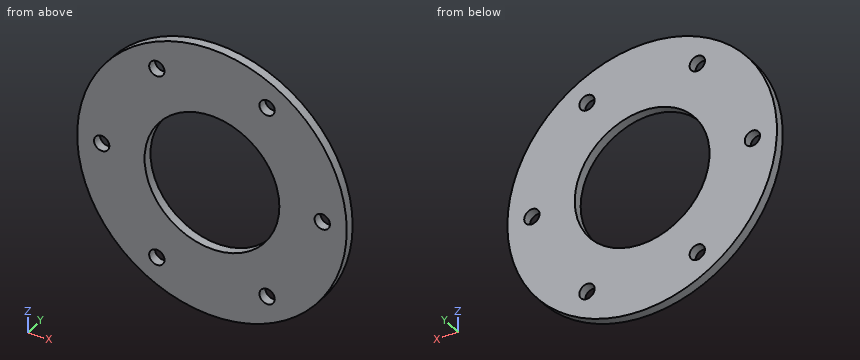
```python
from build123d import *

# Parameters (mm, degrees)
SKETCH1_R           = 139.7
SKETCH1_R_2         = 69.85
BOSS_EXTRUDE1_DEPTH = 9.525
CUT_EXTRUDE1_REACH  = 11.525
SKETCH2_R           = 7.9375


with BuildPart() as part:
    # Sketch1 → Boss-Extrude1 (new body)
    with BuildSketch(Plane(origin=(0, 0, 0), x_dir=(1, 0, 0), z_dir=(0, 1, 0))):
        with Locations((-63.18889636, 128.089070316)):
            Circle(SKETCH1_R)
        with Locations((-63.18889636, 128.089070316)):
            Circle(SKETCH1_R_2, mode=Mode.SUBTRACT)
    extrude(amount=BOSS_EXTRUDE1_DEPTH)

    # Sketch2 → Cut-Extrude1 (cut, up to next)
    with BuildSketch(Plane(origin=(0, 9.525, 0), x_dir=(1, 0, 0), z_dir=(0, 1, 0)), mode=Mode.PRIVATE) as cut_extrude1_sk1:
        with Locations((51.11110364, 128.089070316)):
            Circle(SKETCH2_R)
    cut_extrude1_tool1 = extrude(cut_extrude1_sk1.sketch, amount=-CUT_EXTRUDE1_REACH, mode=Mode.PRIVATE) & part.part
    add(cut_extrude1_tool1.solids().sort_by_distance((51.111104, 9.525, -128.08907))[0], mode=Mode.SUBTRACT)
    # Sketch2 → Cut-Extrude1 (cut, up to next)
    with BuildSketch(Plane(origin=(0, 9.525, 0), x_dir=(1, 0, 0), z_dir=(0, 1, 0)), mode=Mode.PRIVATE) as cut_extrude1_sk2:
        with Locations((-6.03889636, 227.075773969)):
            Circle(SKETCH2_R)
    cut_extrude1_tool2 = extrude(cut_extrude1_sk2.sketch, amount=-CUT_EXTRUDE1_REACH, mode=Mode.PRIVATE) & part.part
    add(cut_extrude1_tool2.solids().sort_by_distance((-6.038896, 9.525, -227.075774))[0], mode=Mode.SUBTRACT)
    # Sketch2 → Cut-Extrude1 (cut, up to next)
    with BuildSketch(Plane(origin=(0, 9.525, 0), x_dir=(1, 0, 0), z_dir=(0, 1, 0)), mode=Mode.PRIVATE) as cut_extrude1_sk3:
        with Locations((-120.33889636, 227.075773969)):
            Circle(SKETCH2_R)
    cut_extrude1_tool3 = extrude(cut_extrude1_sk3.sketch, amount=-CUT_EXTRUDE1_REACH, mode=Mode.PRIVATE) & part.part
    add(cut_extrude1_tool3.solids().sort_by_distance((-120.338896, 9.525, -227.075774))[0], mode=Mode.SUBTRACT)
    # Sketch2 → Cut-Extrude1 (cut, up to next)
    with BuildSketch(Plane(origin=(0, 9.525, 0), x_dir=(1, 0, 0), z_dir=(0, 1, 0)), mode=Mode.PRIVATE) as cut_extrude1_sk4:
        with Locations((-177.48889636, 128.089070316)):
            Circle(SKETCH2_R)
    cut_extrude1_tool4 = extrude(cut_extrude1_sk4.sketch, amount=-CUT_EXTRUDE1_REACH, mode=Mode.PRIVATE) & part.part
    add(cut_extrude1_tool4.solids().sort_by_distance((-177.488896, 9.525, -128.08907))[0], mode=Mode.SUBTRACT)
    # Sketch2 → Cut-Extrude1 (cut, up to next)
    with BuildSketch(Plane(origin=(0, 9.525, 0), x_dir=(1, 0, 0), z_dir=(0, 1, 0)), mode=Mode.PRIVATE) as cut_extrude1_sk5:
        with Locations((-120.33889636, 29.102366663)):
            Circle(SKETCH2_R)
    cut_extrude1_tool5 = extrude(cut_extrude1_sk5.sketch, amount=-CUT_EXTRUDE1_REACH, mode=Mode.PRIVATE) & part.part
    add(cut_extrude1_tool5.solids().sort_by_distance((-120.338896, 9.525, -29.102367))[0], mode=Mode.SUBTRACT)
    # Sketch2 → Cut-Extrude1 (cut, up to next)
    with BuildSketch(Plane(origin=(0, 9.525, 0), x_dir=(1, 0, 0), z_dir=(0, 1, 0)), mode=Mode.PRIVATE) as cut_extrude1_sk6:
        with Locations((-6.03889636, 29.102366663)):
            Circle(SKETCH2_R)
    cut_extrude1_tool6 = extrude(cut_extrude1_sk6.sketch, amount=-CUT_EXTRUDE1_REACH, mode=Mode.PRIVATE) & part.part
    add(cut_extrude1_tool6.solids().sort_by_distance((-6.038896, 9.525, -29.102367))[0], mode=Mode.SUBTRACT)


solid = part.part
```
Here's how the part is built. I have some questions about the finished solid (model axes, mm). Give positions to 0.01 mm unless a question says otherwise; leave off trailing zeros. Order: outer loops, then holes, each group sorted by start corner. A loop starts at its lowest first (then second) coordinate and runs counter-clockwise, first axis right, second up. Notation, with made-up numbers: (86.5, 38.5) - (109.5, 38.5) arc R19 cw to (109.5, 73.5) - close; hole circle Ø4 at (56, -7). An arc over 180 degrees is marked (long way). Answer as a JSON object with one key per item and string values. Group by question number.
Item 1: For P1, Ø14.5, axis at x = -6.04, z = -227.08, coming from the -Y side; P2, Ø2, axis at y = 2.5, z = -51, coming from the -X side; P3, Ø4, axis at x = -159, y = 4, coming from the +Z side; P4, Ø1, axis at y = 3.5, z = -169.5, coming from the -X side, each with a flat end and sliding along its axis, tell me the tip position at first contact or that it passes through.
Item 2: If we section it at B-B on z = -156: Please give me the cut outline in (x, y) (3 decimals).
Item 3: If we section it at C-C on x = -124.5: Please give me the cut outline in (y, z) (3 decimals), and give its area (3 significant figures).
Item 4: If we section it at A-A on x = 52: Please give me the cut outline in (y, z) (1 decimal).
Item 5: If we section it at D-D on y = 5.25: Give the number of separate pieces and of enclosed holes in the cut face, and give its area (3 significant figures).
Item 6: Please list where these lines run through material, in increasing order: probe 1 along Z at (x, y) = (0, 8); probe 2 along Z at (x, y) = (-65.5, 7.5); probe 3 along X at (y, z) = (4.5, -27.5).
Result set:
{
 "1": {"P1": "through", "P2": "x = -180.35", "P3": "z = -24.57", "P4": "x = -196.76"},
 "2": {"outline": "(-200.072, 0) - (-127.22, 0) - (-127.22, 9.525) - (-200.072, 9.525) - close; (0.842, 0) - (73.695, 0) - (73.695, 9.525) - (0.842, 9.525) - close"},
 "3": {"outline": "(0, -253.616) - (9.525, -253.616) - (9.525, -233.835) - (0, -233.835) - close; (0, -220.316) - (9.525, -220.316) - (9.525, -161.555) - (0, -161.555) - close; (0, -94.623) - (9.525, -94.623) - (9.525, -35.862) - (0, -35.862) - close; (0, -22.343) - (9.525, -22.343) - (9.525, -2.562) - (0, -2.562) - close", "area": "1,500 mm²"},
 "4": {"outline": "(0, -207.1) - (9.5, -207.1) - (9.5, -136) - (0, -136) - close; (0, -120.2) - (9.5, -120.2) - (9.5, -49) - (0, -49) - close"},
 "5": {"separate pieces": "1", "enclosed holes": "7", "area": "44,800 mm²"},
 "6": {"probe 1": "-252.68 to -232.23, -221.92 to -157.86, -98.32 to -34.25, -23.95 to -3.5", "probe 2": "-267.77 to -197.9, -58.28 to 11.59", "probe 3": "-160.13 to -128.11, -112.56 to -13.81, 1.74 to 33.75"}
}
